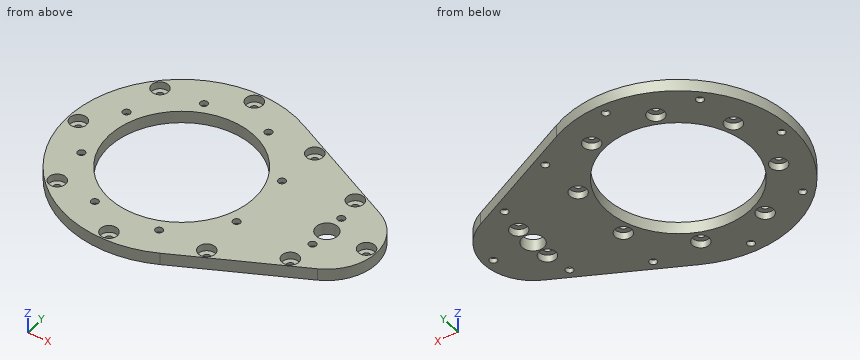
```python
from build123d import *

# Parameters (mm, degrees)
SKETCH1_R           = 1.55
SKETCH1_R_2         = 4.5
SKETCH1_R_3         = 30
BOSS_EXTRUDE2_DEPTH = 5
SKETCH2_R           = 3.5
CUT_EXTRUDE1_DEPTH  = 3
SKETCH3_R           = 3.5
CUT_EXTRUDE2_DEPTH  = 3


with BuildPart() as part:
    # Sketch1 → Boss-Extrude2 (new body)
    with BuildSketch(Plane.XY):
        with BuildLine():
            Line((69.554166667, 18.392174041), (20.855868056, 42.36555049))
            ThreePointArc((20.855868056, 42.36555049), (-47.220833333, 0), (20.855868056, -42.36555049))
            Line((20.855868056, -42.36555049), (69.554166667, -18.392174041))
            ThreePointArc((69.554166667, -18.392174041), (81, 0), (69.554166667, 18.392174041))
        make_face()
        with Locations((60.5, 8.5)):
            Circle(SKETCH1_R, mode=Mode.SUBTRACT)
        with Locations((60.5, -8.5)):
            Circle(SKETCH1_R, mode=Mode.SUBTRACT)
        with Locations((60.5, 0)):
            Circle(SKETCH1_R_2, mode=Mode.SUBTRACT)
        Circle(SKETCH1_R_3, mode=Mode.SUBTRACT)
        with Locations((0, 43)):
            Circle(SKETCH1_R, mode=Mode.SUBTRACT)
        with Locations((-30.405591591, 30.405591591)):
            Circle(SKETCH1_R, mode=Mode.SUBTRACT)
        with Locations((-43, 0)):
            Circle(SKETCH1_R, mode=Mode.SUBTRACT)
        with Locations((-30.405591591, -30.405591591)):
            Circle(SKETCH1_R, mode=Mode.SUBTRACT)
        with Locations((0, -43)):
            Circle(SKETCH1_R, mode=Mode.SUBTRACT)
        with Locations((32.335783638, 13.393920133)):
            Circle(SKETCH1_R, mode=Mode.SUBTRACT)
        with Locations((32.335783638, -13.393920133)):
            Circle(SKETCH1_R, mode=Mode.SUBTRACT)
        with Locations((13.393920133, -32.335783638)):
            Circle(SKETCH1_R, mode=Mode.SUBTRACT)
        with Locations((-13.393920133, -32.335783638)):
            Circle(SKETCH1_R, mode=Mode.SUBTRACT)
        with Locations((-32.335783638, -13.393920133)):
            Circle(SKETCH1_R, mode=Mode.SUBTRACT)
        with Locations((-32.335783638, 13.393920133)):
            Circle(SKETCH1_R, mode=Mode.SUBTRACT)
        with Locations((-13.393920133, 32.335783638)):
            Circle(SKETCH1_R, mode=Mode.SUBTRACT)
        with Locations((13.393920133, 32.335783638)):
            Circle(SKETCH1_R, mode=Mode.SUBTRACT)
        with Locations((32.94935499, 31.953706526)):
            Circle(SKETCH1_R, mode=Mode.SUBTRACT)
        with Locations((58.815707785, 19.220123822)):
            Circle(SKETCH1_R, mode=Mode.SUBTRACT)
        with Locations((32.94935499, -31.953706526)):
            Circle(SKETCH1_R, mode=Mode.SUBTRACT)
        with Locations((58.815707785, -19.220123822)):
            Circle(SKETCH1_R, mode=Mode.SUBTRACT)
        with Locations((77, 0)):
            Circle(SKETCH1_R, mode=Mode.SUBTRACT)
    extrude(amount=BOSS_EXTRUDE2_DEPTH)

    # Sketch2 → Cut-Extrude1 (cut)
    with BuildSketch(Plane(origin=(0, 0, 0), x_dir=(-1, 0, 0), z_dir=(0, 0, -1))):
        with Locations((-60.5, 8.5)):
            Circle(SKETCH2_R)
        with Locations((-60.5, -8.5)):
            Circle(SKETCH2_R)
        with Locations((-13.393920133, 32.335783638)):
            Circle(SKETCH2_R)
        with Locations((13.393920133, 32.335783638)):
            Circle(SKETCH2_R)
        with Locations((32.335783638, 13.393920133)):
            Circle(SKETCH2_R)
        with Locations((32.335783638, -13.393920133)):
            Circle(SKETCH2_R)
        with Locations((13.393920133, -32.335783638)):
            Circle(SKETCH2_R)
        with Locations((-13.393920133, -32.335783638)):
            Circle(SKETCH2_R)
        with Locations((-32.335783638, -13.393920133)):
            Circle(SKETCH2_R)
        with Locations((-32.335783638, 13.393920133)):
            Circle(SKETCH2_R)
    extrude(amount=-CUT_EXTRUDE1_DEPTH, mode=Mode.SUBTRACT)

    # Sketch3 → Cut-Extrude2 (cut)
    with BuildSketch(Plane.XY.offset(5)):
        with Locations((0, 43)):
            Circle(SKETCH3_R)
        with Locations((-30.405591591, 30.405591591)):
            Circle(SKETCH3_R)
        with Locations((-43, 0)):
            Circle(SKETCH3_R)
        with Locations((-30.405591591, -30.405591591)):
            Circle(SKETCH3_R)
        with Locations((0, -43)):
            Circle(SKETCH3_R)
        with Locations((32.94935499, 31.953706526)):
            Circle(SKETCH3_R)
        with Locations((58.815707785, 19.220123822)):
            Circle(SKETCH3_R)
        with Locations((32.94935499, -31.953706526)):
            Circle(SKETCH3_R)
        with Locations((58.815707785, -19.220123822)):
            Circle(SKETCH3_R)
        with Locations((77, 0)):
            Circle(SKETCH3_R)
    extrude(amount=-CUT_EXTRUDE2_DEPTH, mode=Mode.SUBTRACT)


solid = part.part
```
Geometry check sheet. Reference: the model listing, model coordinates, mm. Coordinates: 2 decimals unless noted, no trailing zeros. Loops run counter-clockwise (first coordinate to the right, second up) from the corner with the lowest first, then second, coordinate; pieces in that order, holes last. Notation, with made-up numbers: (28.25, 25.25) - (69.25, 25.25) arc R10 ccw to (69.25, 32.25) - close; hole circle Ø7 at (13, 19). An arc over 180 degrees is marked (long way). One line per item, written item: value. Start each with the question number.
(1) Material ranges on line 1 (X direction, y = -20.5, z = 4.7); line 2 (X direction, y = -12, z = 3.5); line 3 (X direction, y = -17.5, z = 3.95), recorded low to high. Write a range as [from, to].
(2) Cross-section at C-C on x = -43. Enter the section's corners in (y, z).
(3) Cross-section at A-A on x = 0. Enter the section's corners in (y, z), plus the area to 3 significant figures.
(4) Cross-section at B-B on y = 0. Enter the section's corners in (x, z).
(5) Cross-section at D-D on x = 77. Enter the section's corners in (y, z).
(6) Depth check by flat-ended pin: P1, Ø7.5, axis at x = 31.5, y = -32, coming from the +Z side; P2, Ø2, axis at x = -33.5, z = 4, coming from the +Y side; P3, Ø1, axis at x = 65, z = 3.5, coming from the -Y side; P4, Ø1.5, axis at x = 37, z = 2.5, coming from the -Y side. Enter the tip coordinate at first touch or a pass-through.
Results below:
1. line 1: x = [-42.54, -21.9], [21.9, 55.56], [62.07, 65.27]
1. line 2: x = [-45.67, -33.01], [-31.66, -27.5], [27.5, 31.66], [33.01, 77.12]
1. line 3: x = [-43.86, -24.37], [24.37, 55.77], [61.86, 71.18]
2. outline: (-19.51, 0) - (-1.55, 0) - (-1.55, 2) - (-3.5, 2) - (-3.5, 5) - (-19.51, 5) - close; (1.55, 0) - (19.51, 0) - (19.51, 5) - (3.5, 5) - (3.5, 2) - (1.55, 2) - close
3. outline: (-47.22, 0) - (-44.55, 0) - (-44.55, 2) - (-46.5, 2) - (-46.5, 5) - (-47.22, 5) - close; (-41.45, 0) - (-30, 0) - (-30, 5) - (-39.5, 5) - (-39.5, 2) - (-41.45, 2) - close; (30, 0) - (41.45, 0) - (41.45, 2) - (39.5, 2) - (39.5, 5) - (30, 5) - close; (44.55, 0) - (47.22, 0) - (47.22, 5) - (46.5, 5) - (46.5, 2) - (44.55, 2) - close
3. area: 118 mm2
4. outline: (-47.22, 0) - (-44.55, 0) - (-44.55, 2) - (-46.5, 2) - (-46.5, 5) - (-47.22, 5) - close; (-41.45, 0) - (-30, 0) - (-30, 5) - (-39.5, 5) - (-39.5, 2) - (-41.45, 2) - close; (30, 0) - (56, 0) - (56, 5) - (30, 5) - close; (65, 0) - (75.45, 0) - (75.45, 2) - (73.5, 2) - (73.5, 5) - (65, 5) - close; (78.55, 0) - (81, 0) - (81, 5) - (80.5, 5) - (80.5, 2) - (78.55, 2) - close
5. outline: (-12.17, 0) - (-1.55, 0) - (-1.55, 2) - (-3.5, 2) - (-3.5, 5) - (-12.17, 5) - close; (1.55, 0) - (12.17, 0) - (12.17, 5) - (3.5, 5) - (3.5, 2) - (1.55, 2) - close
6. P1: stops at z = 5
6. P2: stops at y = 34.26
6. P3: stops at y = -20.88
6. P4: stops at y = -34.79
